For this review, take the finished solid that the model builds, in its own axes (mm). A direction names the side the tool comes from. Round coordinates to 2 decimals unless told otherwise and drop trailing zeros. Order: outer loops, then holes, each group sorted by start corner. A loop starts at its lowest first (then second) coordinate and runs counter-clockwise, first axis right, second up. Notation, with made-up numbers: (56.5, 47.5) - (83.5, 47.5) arc R17 cw to (83.5, 74.5) - close; hole circle Ø1 at (52.25, -21.5). An arc over 180 degrees is marked (long way). One line per item, written item: value.
```python
from build123d import *

# Parameters (mm, degrees)
F2_R = 1
F3_R = 2


with BuildPart() as f1:
    # F0 (on Front) → F1 (revolve)
    with BuildSketch(Plane.XZ):
        Polygon((17, 69.5), (0, 69.5), (0, -69.5), (4, -57.5), (4, 29.5), (8, 29.5), (8, 39.5), (8, 61.5), (17, 61.5), align=None)
    revolve(axis=Axis((0, 0, 0), (0, 0, -1)))

    # F2
    f2_edges = [f1.edges().sort_by_distance(p)[0] for p in [
        (-17, 0, 69.5),
        (-17, 0, 61.5),
        (-8, 0, 29.5),
    ]]
    fillet(f2_edges, radius=F2_R)

    # F3
    f3_edges = [f1.edges().sort_by_distance(p)[0] for p in [
        (-8, 0, 61.5),
        (-4, 0, 29.5),
    ]]
    fillet(f3_edges, radius=F3_R)


solid = f1.part
```
Item 1: Machinability: for faces 1 (the flat face through (0, 0, 69.5)), 2 (the flat face through (-6, -2, 29.5)), which of the approach directions +Z, -Z, +X, -X, +Y, -Y give a long, thin tool a straight path to every point of the face, cutting with its end or side? Answer none if there is none.
Returned:
face 1: +Z, +X, -X, +Y, -Y
face 2: -Z
Item 2: Wall thickness on line 1 (Z direction, x = 11, y = -5); line 2 (Z direction, x = 6, y = -2); line 3 (X direction, y = -1, z = 57): over which ranges is each line inside the solid? List them lowest first.
Returned:
line 1: 61.5 to 69.5
line 2: 29.5 to 69.5
line 3: -7.94 to 7.94
Item 3: Take a section at A-A (z = 15.5). Write out the cut boundary in (x, y), plus the area to 3 significant figures.
Returned:
outline: circle Ø8 at (0, 0)
area: 50.3 mm^2
Item 4: For P1, Ø1, axis at x = -13, y = -1, coming from the -Z side; P2, Ø5, axis at x = 1.5, z = 44.5, coming from the +Y side; P3, Ø1, axis at y = -1.5, z = -26.5, coming from the +X side; P4, Ø1.5, axis at x = 6.5, z = 2.5, coming from the +Y side, all flat-tipped, find the tip position at first contact; note any pin that passes through.
Returned:
P1: z = 61.5
P2: y = 8
P3: x = 3.87
P4: through
